Part model, mm, in its own coordinate system. A direction names the side the tool comes from. Coordinates: 2 decimals unless noted, no trailing zeros. Loops run counter-clockwise (first coordinate to the right, second up) from the corner with the lowest first, then second, coordinate; pieces in that order, holes last. Notation, with made-up numbers: (87, 57.25) - (122, 57.25) arc R22 cw to (122, 83.25) - close; hole circle Ø8 at (60.25, 62). An arc over 180 degrees is marked (long way). Use a Markdown table: item, result. Add a question column.
1. Pull direction Z, two halves, no side cores. Call faces 6 (the flat face through (31, 11.296, 167)), 7 (the cylindrical face through (99.15, 34.04, 132.88)), 8 (the flat face through (73, 2, 0)): pulls with the +Z half, pulls with the -Z half, needs draft (parallel to the pull), parting line crosses it, or undercut.
2. Wall check: probe 1 along Y at (x, z) = (43, 47.5); probe 2 along Z at (x, y) = (8.5, 33); probe 3 along X at (y, z) = (15.5, 68.5). Give the ranges that are in metal, low to high. Write a range as [from, to].
3. Band-saw the part on C-C, the plane y = 19. Give the cut face in (x, z), plus the area to 3 significant figures.
4. Band-saw the part on B-B, the plane z = 78. Give the cut face in (x, y).
5. Band-saw the part on D-D, the plane z = 161.5. Give the cut face in (x, y).
6. Band-saw the part on A-A, the plane x = 83. Give the cut face in (y, z), plus the area to 3 significant figures.
7. Drop flat-ended pins along their axis: pin 1 (4 mm diameter, centred on x = 82.5, z = 24.5, fed in from +Y); pin 2 (8 mm diameter, centred on y = 4, z = 175, fed in from -X); pin 3 (1.5 mm diameter, centred on y = 34.5, z = 32, fed in from -X); pin 4 (2.5 mm diameter, centred on x = 153.5, y = 34.5, fed in from +Z). Give the stop position or say it passes through.
8. 3-axis set-ups, long thin cutter, end or side, ignore diameter. For faces 1 (the flat face through (15, 26.892, 177)), 2 (the flat face through (31, 8.296, 170)), 3 (the flat face through (13.03, 17, 170)), 4 (the flat face through (170, 18, 68)), 5 (the flat face through (49.391, 17, 170)): which of +Z, -Z, +X, -X, +Y, -Y reach the whole face in a straight line?
from build123d import *

# Parameters (mm, degrees)
SKETCH1_W           = 173
SKETCH1_H           = 35.519872746
BOSS_EXTRUDE2_DEPTH = 140
SHELL3_T            = -3
SKETCH3_R           = 6
SKETCH3_R_2         = 3.7
SKETCH3_W           = 99.5
SKETCH3_H           = 23.7
SKETCH3_W_2         = 5.9
SKETCH3_H_2         = 12.3
SKETCH3_W_3         = 5.800374035
SKETCH3_H_3         = 4.8
SKETCH3_W_4         = 5.5
SKETCH3_H_4         = 4.647872836
CUT_EXTRUDE3_DEPTH  = 7.5
SKETCH5_W           = 36.361516307
SKETCH5_H           = 18.595843956
BOSS_EXTRUDE4_DEPTH = 60
SHELL5_START        = 140
SHELL5_OUTLINE_W    = 30.361516307
SHELL5_OUTLINE_H    = 15.595843956
SHELL5_DEPTH        = 57
SKETCH8_W           = 30.361516307
SKETCH8_H           = 14.422474908
CUT_EXTRUDE6_DEPTH  = 20.5


# Read off the part's stored shape, not the designer's step: Shell5
with BuildPart() as part:
    # Sketch1 → Boss-Extrude2 (new body)
    with BuildSketch(Plane.XY):
        with Locations((86.5, 17.759936373)):
            Rectangle(SKETCH1_W, SKETCH1_H)
    extrude(amount=BOSS_EXTRUDE2_DEPTH)

    # Shell3
    shell3_openings = [part.faces().sort_by_distance(p)[0] for p in [
        (86.5, 17.759936373, 0),
    ]]
    offset(amount=SHELL3_T, openings=shell3_openings, kind=Kind.INTERSECTION)

    # Sketch3 → Cut-Extrude3 (cut)
    with BuildSketch(Plane(origin=(0, 35.519872746, 0), x_dir=(1, 0, 0), z_dir=(0, 1, 0))):
        with Locations(Location((39.736956851, -109.200672262, 0), (0, 0, 270))):
            Circle(SKETCH3_R)
        with Locations(Location((100.567495644, -129.464431968, 0), (0, 0, 270))):
            Circle(SKETCH3_R_2)
        with Locations((88.25, -29.85)):
            Rectangle(SKETCH3_W, SKETCH3_H)
        with Locations((28.45, -62.785125048)):
            Rectangle(SKETCH3_W_2, SKETCH3_H_2)
        with Locations((9.910075314, -86.290425048)):
            Rectangle(SKETCH3_W_3, SKETCH3_H_3)
        with Locations((154.184914317, -101.481582974)):
            Rectangle(SKETCH3_W_4, SKETCH3_H_4)
    extrude(amount=-CUT_EXTRUDE3_DEPTH, mode=Mode.SUBTRACT)

    # Sketch5 → Boss-Extrude4 (add)
    with BuildSketch(Plane.XY.offset(140)):
        with Locations((31.210571096, 17.593902052)):
            Rectangle(SKETCH5_W, SKETCH5_H)
    extrude(amount=BOSS_EXTRUDE4_DEPTH)

    # Shell5 outline → Shell5 (cut)
    with BuildSketch(Plane.XY.offset(SHELL5_START)):
        with Locations((31.210571096, 19.093902052)):
            Rectangle(SHELL5_OUTLINE_W, SHELL5_OUTLINE_H)
    extrude(amount=SHELL5_DEPTH, mode=Mode.SUBTRACT)

    # Sketch8 → Cut-Extrude6 (cut)
    with BuildSketch(Plane.XY.offset(140)):
        with Locations((31.210571096, 18.507217528)):
            Rectangle(SKETCH8_W, SKETCH8_H)
    extrude(amount=-CUT_EXTRUDE6_DEPTH, mode=Mode.SUBTRACT)


solid = part.part
Geometry check:
| question | item | result |
|---|---|---|
| 1 | face 6 | needs draft |
| 1 | face 7 | undercut |
| 1 | face 8 | pulls with the -Z half |
| 2 | probe 1 | y = [0, 3], [32.52, 35.52] |
| 2 | probe 2 | z = [0, 83.89], [88.69, 140] |
| 2 | probe 3 | x = [0, 3], [170, 173] |
| 3 | outline | (0, 0) - (3, 0) - (3, 137) - (16.03, 137) - (16.03, 197) - (46.39, 197) - (46.39, 137) - (170, 137) - (170, 0) - (173, 0) - (173, 140) - (49.39, 140) - (49.39, 200) - (13.03, 200) - (13.03, 140) - (0, 140) - close |
| 3 | area | 1,700 mm^2 |
| 4 | outline | (0, 0) - (173, 0) - (173, 35.52) - (0, 35.52) - close; hole (3, 3) - (170, 3) - (170, 32.52) - (3, 32.52) - close |
| 5 | outline | (13.03, 8.3) - (49.39, 8.3) - (49.39, 26.89) - (46.39, 26.89) - (46.39, 11.3) - (16.03, 11.3) - (16.03, 26.89) - (13.03, 26.89) - close |
| 6 | outline | (0, 0) - (3, 0) - (3, 137) - (32.52, 137) - (32.52, 41.7) - (35.52, 41.7) - (35.52, 140) - (0, 140) - close; (32.52, 0) - (35.52, 0) - (35.52, 18) - (32.52, 18) - close |
| 6 | area | 857 mm^2 |
| 7 | pin 1 | stops at y = 3 |
| 7 | pin 2 | passes through |
| 7 | pin 3 | stops at x = 0 |
| 7 | pin 4 | stops at z = 140 |
| 8 | face 1 | +Z, +X, -X, +Y |
| 8 | face 2 | +Z, +X, -X, -Y |
| 8 | face 3 | +Z, -X, +Y, -Y |
| 8 | face 4 | -Z |
| 8 | face 5 | +Z, +X, +Y, -Y |
